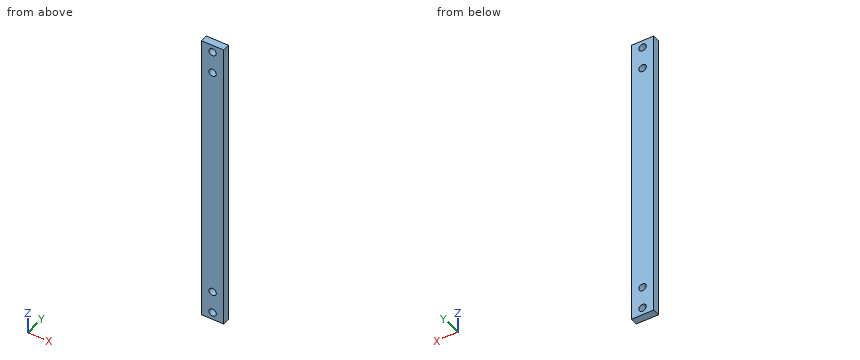
Autodesk Inventor part; units mm, degrees
ref_plane "YZ Plane" through (0, 0, 0) normal (1, 0, 0) x (0, 1, 0)
ref_plane "XZ Plane" through (0, 0, 0) normal (0, 1, 0) x (-1, 0, 0)
ref_plane "XY Plane" through (0, 0, 0) normal (0, 0, 1) x (1, 0, 0)
sketch "Sketch1" plane through (0, 0, 0) normal (0, 1, 0) x (-1, 0, 0)
  line L0 (-3, 40) -> (3, 40)
  line L1 (3, 40) -> (3, -40)
  line L2 (3, -40) -> (-3, -40)
  line L3 (-3, -40) -> (-3, 40)
  circle A0 centre (0, 38) radius 1
  circle A1 centre (0, 32) radius 1
  circle A2 centre (0, -32) radius 1
  circle A3 centre (0, -38) radius 1
  point P0 (0, 0)
extrude "Extrusion1" add sketch "Sketch1" along normal blind 2
properties part number "camera_arm"
Check sheet for the modelled part. Datum: model origin and axes. Units: mm. Give positions to 0.01 mm unless a question says otherwise; leave off trailing zeros. Loops run counter-clockwise (first coordinate to the right, second up) from the corner with the lowest first, then second, coordinate; pieces in that order, holes last. Notation, with made-up numbers: M 65,-8.75 L 101,-8.75 A17 ccw 101,19.25 Z; hole C 85.5,-26 d11. An arc over 180 degrees is marked long. Answer as a JSON object with one key per item and string values. Group by question number.
Q1. Material ranges on line 1 along Z through (x, y) = (0, 1.25); line 2 along Z through (x, y) = (-0.8, 1.55), recorded low to high. Write a range as [from, to].
Q2. Cross-section at C-C on y = 1.3. Record the cut outline in (x, z).
Q3. Go/stop test with flat-tipped pins: P1, Ø1.8, axis at x = 0, z = -38, coming from the -Y side; P2, Ø2.5, axis at x = 0, z = -32, coming from the -Y side. Record where each tip stops, or that it passes through.
Q4. Cross-section at A-A on z = -32. Record the cut outline in (x, y), then the cut area to 3 significant figures.
Q5. Cross-section at B-B on x = 0. Record the cut outline in (y, z).
Evaluation:
{
 "1": {"line 1": "z = [-40, -39], [-37, -33], [-31, 31], [33, 37], [39, 40]", "line 2": "z = [-40, -38.6], [-37.4, -32.6], [-31.4, 31.4], [32.6, 37.4], [38.6, 40]"},
 "2": {"outline": "M -3,-40 L 3,-40 L 3,40 L -3,40 Z; hole C 0,-38 d2; hole C 0,-32 d2; hole C 0,32 d2; hole C 0,38 d2"},
 "3": {"P1": "passes through", "P2": "stops at y = 0"},
 "4": {"outline": "M -3,0 L -1,0 L -1,2 L -3,2 Z; M 1,0 L 3,0 L 3,2 L 1,2 Z", "area": "8.00 mm2"},
 "5": {"outline": "M 0,-40 L 2,-40 L 2,-39 L 0,-39 Z; M 0,-37 L 2,-37 L 2,-33 L 0,-33 Z; M 0,-31 L 2,-31 L 2,31 L 0,31 Z; M 0,33 L 2,33 L 2,37 L 0,37 Z; M 0,39 L 2,39 L 2,40 L 0,40 Z"}
}
